The listing builds one solid part. Answer for the finished solid, in the listing's coordinates (mm). Face numbers are marked on the shaded views. Give positions to 0.01 mm unless a question says otherwise; leave off trailing zeros. Order: outer loops, then holes, each group sorted by start corner. A loop starts at its lowest first (then second) coordinate and runs counter-clockwise, first axis right, second up. Notation, with made-up numbers: (24.25, -9.75) -> (50.25, -9.75) arc R13 cw to (50.25, 5.25) -> close; hole circle Ø11 at (22, 45.25). An arc over 180 degrees is marked (long way). One line per question, with ' | ' between items. Start each with the question number.
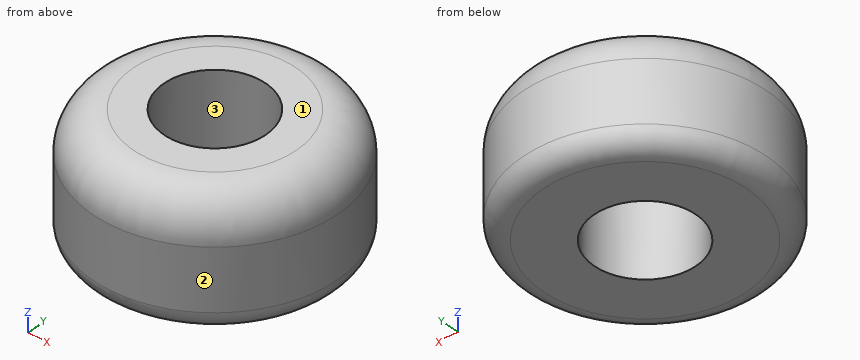
```python
from build123d import *

# Parameters (mm, degrees)
F1_R     = 6
F1_R_2   = 2.5
F2_DEPTH = 6
F3_R     = 2
F4_R     = 1


with BuildPart() as f2:
    # F1 (on face) → F2 (new body)
    with BuildSketch(Plane.XY):
        Circle(F1_R)
        Circle(F1_R_2, mode=Mode.SUBTRACT)
    extrude(amount=F2_DEPTH)

    # F3
    f3_edges = [f2.edges().sort_by_distance(p)[0] for p in [
        (-6, 0, 6),
    ]]
    fillet(f3_edges, radius=F3_R)

    # F4
    f4_edges = [f2.edges().sort_by_distance(p)[0] for p in [
        (-6, 0, 0),
    ]]
    fillet(f4_edges, radius=F4_R)


solid = f2.part
```
(1) Determine the mould class of the marked faces 1, 2 and 3 for opening direction X: pulls with the +X half, pulls with the -X half, needs draft (parallel to the pull), parting line crosses it, or undercut.
(2) The part is cut by section C-C on z = 3.2. Determine the outline of the cut face in (x, y), plus the area to 3 significant figures.
(3) Given P1, Ø3, axis at x = -4, z = 1.5, coming from the +Y side; P2, Ø1.5, axis at y = -1, z = 3.5, coming from the -X side; P3, Ø2, axis at x = -4, z = 5, coming from the -Y side, each flat-ended and moving along its own axis, determine where each tip first touches the part or whether it passes through.
(4) The part is cut by section A-A on x = 0. Determine the outline of the cut face in (y, z), plus the area to 3 significant figures.
(5) Consider line 1 (Y direction, x = 0, z = 3.6); line 2 (Y direction, x = 0, z = 4.45); line 3 (Z direction, x = 1, y = 4). Determine where each line is inside the solid, lowest interval first.
(6) The part is cut by section D-D on z = 5.65. Determine the outline of the cut face in (x, y), plus the area to 3 significant figures.
Result sheet:
1) face 1: needs draft | face 2: parting line crosses it | face 3: undercut
2) outline: circle Ø12 at (0, 0); hole circle Ø5 at (0, 0) | area: 93.5 mm^2
3) P1: stops at y = 5.45 | P2: stops at x = -5.99 | P3: stops at y = -5.04
4) outline: (-6, 1) arc R1 ccw to (-5, 0) -> (-2.5, 0) -> (-2.5, 6) -> (-4, 6) arc R2 ccw to (-6, 4) -> close; (2.5, 0) -> (5, 0) arc R1 ccw to (6, 1) -> (6, 4) arc R2 ccw to (4, 6) -> (2.5, 6) -> close | area: 39.9 mm^2
5) line 1: y = -6 to -2.5, 2.5 to 6 | line 2: y = -5.95 to -2.5, 2.5 to 5.95 | line 3: z = 0 to 6
6) outline: circle Ø10.26 at (0, 0); hole circle Ø5 at (0, 0) | area: 63.1 mm^2
